The model under review builds one solid part; all positions refer to its coordinate system, in mm. Give positions to 0.01 mm unless a question says otherwise; leave off trailing zeros. Order: outer loops, then holes, each group sorted by start corner. A loop starts at its lowest first (then second) coordinate and runs counter-clockwise, first axis right, second up.
```python
from build123d import *

# Parameters (mm, degrees)
F0_R     = 2.54
F1_DEPTH = 63.5
F2_R     = 0.508
F3_SIZE  = 2.286


with BuildPart() as f1:
    # F0 (on Front) → F1 (new body)
    with BuildSketch(Plane.XZ):
        with Locations((-11.582997, 5.600415)):
            Circle(F0_R)
    extrude(amount=F1_DEPTH)

    # F2
    f2_edges = [f1.edges().sort_by_distance(p)[0] for p in [
        (-14.122997, 0, 5.600415),
    ]]
    fillet(f2_edges, radius=F2_R)

    # F3
    f3_edges = [f1.edges().sort_by_distance(p)[0] for p in [
        (-14.122997, -63.5, 5.600415),
    ]]
    chamfer(f3_edges, length=F3_SIZE)


solid = f1.part
```
Item 1: Take a section at A-A (y = -42). Give the boundary of the cut face in (x, z).
Values found:
outline: circle Ø5.08 at (-11.58, 5.6)
Item 2: For line 1 (Z direction, x = -11.5, y = -27); line 2 (X direction, y = -21, z = 5.4); line 3 (X direction, y = -23.5, z = 3.65), list the stretches that pass through material, from the lowest coordinate up.
Values found:
line 1: z = 3.06 to 8.14
line 2: x = -14.12 to -9.05
line 3: x = -13.21 to -9.96
Item 3: Clearance check with flat-ended pins moving along their axes: pin 1 Ø1 at (x, z) = (-13, 5.5) entering from +Y; pin 2 Ø2 at (y, z) = (-45.5, 7) entering from +X; pin 3 Ø1 at (x, y) = (-12.5, -42) entering from +Z. State where each tip first meets the part, or that it passes through.
Values found:
pin 1: stops at y = 0
pin 2: stops at x = -9.07
pin 3: stops at z = 8.11
